```python
from build123d import *

# Parameters (mm, degrees)
F0_R     = 110
F0_R_2   = 90
F1_DEPTH = 25.4
F4_R     = 3
F5_DEPTH = 110.5
F7_R     = 5
F8_DEPTH = 25.5


with BuildPart() as f1:
    # F0 (on Right) → F1 (new body)
    with BuildSketch(Plane.YZ):
        Circle(F0_R)
        Circle(F0_R_2, mode=Mode.SUBTRACT)
    extrude(amount=-F1_DEPTH)

    # F4 (on face) → F5 (cut, symmetric)
    with BuildSketch(Plane(origin=(0, 0, 0), x_dir=(-1, 0, 0), z_dir=(0, 0.707107, -0.707107))):
        with Locations((12.223506, 0)):
            Circle(F4_R)
    extrude(amount=F5_DEPTH, both=True, mode=Mode.SUBTRACT)

    # F7 (on face) → F8 (cut)
    with BuildSketch(Plane.YZ):
        with Locations((0, 96.278802)):
            Circle(F7_R)
        with Locations((-96.278802, 0)):
            Circle(F7_R)
        with Locations((0, -96.278802)):
            Circle(F7_R)
        with Locations((96.278802, 0)):
            Circle(F7_R)
    extrude(amount=-F8_DEPTH, mode=Mode.SUBTRACT)


solid = f1.part
```
Can you work these out from the model? Positions are in its coordinate system, mm. Coordinates: 2 decimals unless noted, no trailing zeros. Order: outer loops, then holes, each group sorted by start corner. A loop starts at its lowest first (then second) coordinate and runs counter-clockwise, first axis right, second up. Notation, with made-up numbers: (72, 9.5) - (76, 9.5) arc R20 ccw to (76, 36.5) - close; hole circle Ø7 at (58.5, 53). An arc over 180 degrees is marked (long way). Answer in a Markdown table with one row per item.
1. Suppose I cut it at D-D (z = 52.5). Please give me the cut outline in (x, y).
Reply:
| item | result |
|---|---|
| outline | (-25.4, -96.66) - (0, -96.66) - (0, -73.1) - (-25.4, -73.1) - close; (-25.4, 73.1) - (0, 73.1) - (0, 96.66) - (-25.4, 96.66) - close |
2. For pin 1 (4 mm diameter, centred on x = -12, z = 33.5, fed in from -Y); pin 2 (1.5 mm diameter, centred on x = -9, z = -6, fed in from +Y); pin 3 (1 mm diameter, centred on x = -9, z = -61, fed in from -Y); pin 4 (11.5 mm diameter, centred on y = 0, z = 96.28, fed in from -X), each with a flat end and sliding along its axis, tell me the tip position at first contact or that it passes through.
Reply:
| item | result |
|---|---|
| pin 1 | stops at y = -105.39 |
| pin 2 | stops at y = 109.87 |
| pin 3 | stops at y = -91.87 |
| pin 4 | stops at x = -25.4 |
3. Suppose I cut it at A-A (y = 0). Please give me the cut outline in (x, z), and give its area (3 significant figures).
Reply:
| item | result |
|---|---|
| outline | (-25.4, -110) - (0, -110) - (0, -101.28) - (-25.4, -101.28) - close; (-25.4, -91.28) - (0, -91.28) - (0, -90) - (-25.4, -90) - close; (-25.4, 90) - (0, 90) - (0, 91.28) - (-25.4, 91.28) - close; (-25.4, 101.28) - (0, 101.28) - (0, 110) - (-25.4, 110) - close |
| area | 508 mm^2 |
4. If we mould it in two halves opening along X, with no side actions, what happens to faces 1 (the flat face through (0, -17, -89)), 2 (the cylindrical face through (-13.836, 72.581, -69.003)), 3 (the cylindrical face through (-12.522, 91.284, 0.22)), 4 (the flat face through (-25.4, -17, -89))? For each: pulls with the +X half, pulls with the -X half, needs draft (parallel to the pull), parting line crosses it, or undercut.
Reply:
| item | result |
|---|---|
| face 1 | pulls with the +X half |
| face 2 | undercut |
| face 3 | needs draft |
| face 4 | pulls with the -X half |
5. If I drill on line 1 along Z through (x, y) = (-18.25, 0); line 2 along Y through (x, z) = (-4.5, -31.5); line 3 along Z through (x, y) = (-21.75, -51), over which ranges is the centre line in solid material (lowest first)?
Reply:
| item | result |
|---|---|
| line 1 | z = -110 to -101.28, -91.28 to -90, 90 to 91.28, 101.28 to 110 |
| line 2 | y = -105.39 to -84.31, 84.31 to 105.39 |
| line 3 | z = -97.46 to -74.16, 74.16 to 97.46 |
6. Suppose I cut it at C-C (x = -17.75). Please give me the cut outline in (y, z).
Reply:
| item | result |
|---|---|
| outline | circle Ø220 at (0, 0); hole circle Ø10 at (-96.28, 0); hole circle Ø180 at (0, 0); hole circle Ø10 at (0, -96.28); hole circle Ø10 at (0, 96.28); hole circle Ø10 at (96.28, 0) |
